Check sheet for the modelled part. Datum: model origin and axes. Units: mm. Face numbers are marked on the shaded views. A direction names the side the tool comes from. Round coordinates to 2 decimals unless told otherwise and drop trailing zeros. Order: outer loops, then holes, each group sorted by start corner. A loop starts at its lowest first (then second) coordinate and runs counter-clockwise, first axis right, second up.
```python
from build123d import *

# Parameters (mm, degrees)
SKETCH2_W               = 20
SKETCH2_H               = 50
BOSS_EXTRUDE1_DEPTH     = 22.5
SKETCH3_W               = 5
SKETCH3_H               = 40
BOSS_EXTRUDE2_DEPTH     = 40
SKETCH4_R               = 7.5
CUT_EXTRUDE1_DEPTH      = 23.5
CUT_EXTRUDE1_DEPTH_BACK = 23.5


with BuildPart() as part:
    # Sketch2 → Boss-Extrude1 (new body, symmetric)
    with BuildSketch(Plane(origin=(0, 0, 0), x_dir=(0, 0, -1), z_dir=(1, 0, 0))):
        Rectangle(SKETCH2_W, SKETCH2_H)
    extrude(amount=BOSS_EXTRUDE1_DEPTH, both=True)

    # Sketch3 → Boss-Extrude2 (add)
    with BuildSketch(Plane.XY.offset(10)):
        with Locations((-20, -23)):
            Rectangle(SKETCH3_W, SKETCH3_H)
    extrude(amount=BOSS_EXTRUDE2_DEPTH)

    # Sketch4 → Cut-Extrude1 (cut, two sides)
    with BuildSketch(Plane(origin=(0, 0, 0), x_dir=(0, 0, -1), z_dir=(1, 0, 0))) as cut_extrude1_sk:
        with Locations((0, -15)):
            Circle(SKETCH4_R)
        with Locations((0, 15)):
            Circle(SKETCH4_R)
    extrude(amount=CUT_EXTRUDE1_DEPTH, mode=Mode.SUBTRACT)
    extrude(cut_extrude1_sk.sketch, amount=-CUT_EXTRUDE1_DEPTH_BACK, mode=Mode.SUBTRACT)


solid = part.part
```
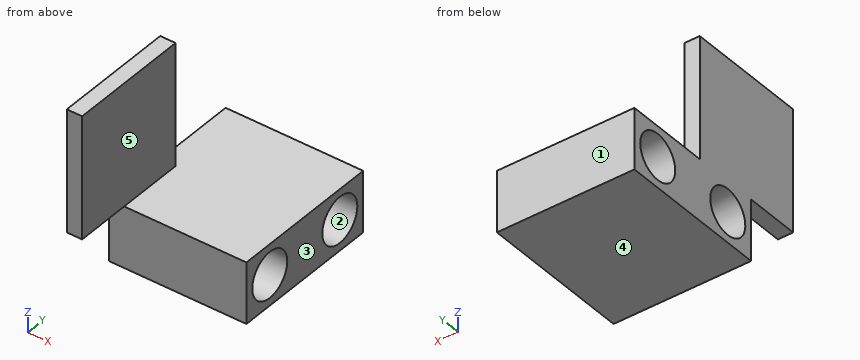
Item 1: Release check for a two-part mould opening along Y. For the marked faces 1, 2 and 3 record: released by +Y, released by -Y, zero draft, split by the parting line, or undercut.
Answer:
face 1: released by +Y
face 2: undercut
face 3: zero draft
Item 2: Sectioned sample at A-A (y = -15). Record the cut outline in (x, z).
Answer:
outline: (-22.5, -10) - (22.5, -10) - (22.5, -7.5) - (-22.5, -7.5) - close; (-22.5, 7.5) - (22.5, 7.5) - (22.5, 10) - (-17.5, 10) - (-17.5, 50) - (-22.5, 50) - close
Item 3: Go/stop test with flat-tipped pins: P1, Ø4, axis at x = -20.5, z = 38.5, coming from the +Y side; P2, Ø20, axis at y = -32, z = 35.5, coming from the +X side; P3, Ø12, axis at x = -4.5, z = 5.5, coming from the -Y side. Record where each tip stops, or that it passes through.
Answer:
P1: stops at y = -3
P2: stops at x = -17.5
P3: stops at y = -25
Item 4: Sectioned sample at C-C (x = 17). Record the cut outline in (y, z).
Answer:
outline: (-25, -10) - (25, -10) - (25, 10) - (-25, 10) - close; hole circle Ø15 at (-15, 0); hole circle Ø15 at (15, 0)
Item 5: Access from +Z, -Z, +X, -X, +Y, -Y to the whole of each face (thin tool, end or side, straight path). Record for the marked faces 4 and 5.
Answer:
face 4: -Z, +X, -X, +Y, -Y
face 5: +Z, +X, +Y, -Y
Item 6: Sectioned sample at D-D (y = 15). Record the cut outline in (x, z).
Answer:
outline: (-22.5, -10) - (22.5, -10) - (22.5, -7.5) - (-22.5, -7.5) - close; (-22.5, 7.5) - (22.5, 7.5) - (22.5, 10) - (-22.5, 10) - close
Item 7: Sectioned sample at B-B (z = 0). Record the cut outline in (x, y).
Answer:
outline: (-22.5, -25) - (22.5, -25) - (22.5, -22.5) - (-22.5, -22.5) - close; (-22.5, -7.5) - (22.5, -7.5) - (22.5, 7.5) - (-22.5, 7.5) - close; (-22.5, 22.5) - (22.5, 22.5) - (22.5, 25) - (-22.5, 25) - close
Item 8: Scan lines: line 1 along Y through (x, z) = (-9, 0); line 2 along Z through (x, y) = (-2.5, 15); line 3 along Y through (x, z) = (-6.5, 6). Record each from-to range of solid material in increasing order.
Answer:
line 1: y = -25 to -22.5, -7.5 to 7.5, 22.5 to 25
line 2: z = -10 to -7.5, 7.5 to 10
line 3: y = -25 to -19.5, -10.5 to 10.5, 19.5 to 25
